from build123d import *

# Parameters (mm, degrees)
SKETCH3_W           = 57.15
SKETCH3_H           = 6.35
BOSS_EXTRUDE2_DEPTH = 50.8
SKETCH4_R           = 5.05
SKETCH4_R_2         = 4.7625
SKETCH4_R_3         = 1.5
SKETCH4_R_4         = 1.984375
CUT_EXTRUDE1_DEPTH  = 6.35


with BuildPart() as part:
    # Sketch3 → Boss-Extrude2 (new body)
    with BuildSketch(Plane.XY):
        with Locations((-92.644673345, -3.175)):
            Rectangle(SKETCH3_W, SKETCH3_H)
    extrude(amount=BOSS_EXTRUDE2_DEPTH)

    # Sketch4 → Cut-Extrude1 (cut)
    with BuildSketch(Plane(origin=(0, 0, 0), x_dir=(1, 0, 0), z_dir=(0, 1, 0))):
        with Locations((-108.519673345, -25.4)):
            Circle(SKETCH4_R)
        with Locations((-79.944673345, -38.1)):
            Circle(SKETCH4_R_2)
        with Locations((-108.519673345, -17.27)):
            Circle(SKETCH4_R_3)
        with Locations((-87.802397451, -30.242275894)):
            Circle(SKETCH4_R_4)
        with Locations((-72.086949239, -30.242275894)):
            Circle(SKETCH4_R_4)
        with Locations((-72.086949239, -45.957724106)):
            Circle(SKETCH4_R_4)
        with Locations((-87.802397451, -45.957724106)):
            Circle(SKETCH4_R_4)
        with Locations((-116.649673345, -25.4)):
            Circle(SKETCH4_R_3)
        with Locations((-100.389673345, -25.4)):
            Circle(SKETCH4_R_3)
        with Locations((-108.519673345, -33.53)):
            Circle(SKETCH4_R_3)
        with Locations((-87.802397451, -4.842275894)):
            Circle(SKETCH4_R_4)
        with Locations((-72.086949239, -4.842275894)):
            Circle(SKETCH4_R_4)
        with Locations((-72.086949239, -20.557724106)):
            Circle(SKETCH4_R_4)
        with Locations((-87.802397451, -20.557724106)):
            Circle(SKETCH4_R_4)
        with Locations((-79.944673345, -12.7)):
            Circle(SKETCH4_R_2)
    extrude(amount=-CUT_EXTRUDE1_DEPTH, mode=Mode.SUBTRACT)


solid = part.part
The model under review builds one solid part; all positions refer to its coordinate system, in mm. Round coordinates to 2 decimals unless told otherwise and drop trailing zeros. Write each loop counter-clockwise with the first axis right and the second up, starting at its lowest first coordinate (ties: lowest second). Pieces come first, ordered by that corner, then holes. Notation, with made-up numbers: (25.5, 37) - (84.5, 37) arc R19 cw to (84.5, 48) - close; hole circle Ø2 at (19.25, -17.75). An arc over 180 degrees is marked (long way). One line per item, written item: value. Start each with the question number.
1. Clearance check with flat-ended pins moving along their axes: P1, Ø5, axis at x = -87.8, z = 30.24, coming from the +Y side; P2, Ø3.5, axis at x = -87.8, z = 45.96, coming from the -Y side. State where each tip first meets the part, or that it passes through.
2. Consider section A-A on z = 12.7. Write out the cut boundary in (x, y), and give its area (3 significant figures).
3. The part is to be moulded in two halves that separate along Z. For faces 1 (the face through (-121.22, -3, 25)), 2 (the face through (-93, -3, 50.8)), 3 (the face through (-85.97, -3.13, 46.72)), say which applies: released by +Z, released by -Z, zero draft, split by the parting line, or undercut.
4. Consider section C-C on x = -89. Write out the cut boundary in (y, z).
5. Consider section B-B on z = 25.4. Write out the cut boundary in (x, y), and give its area (3 significant figures).
6. To check wall thickness, follow L1, parallel to X at y = -2.5, z = 25.4; L2, parallel to X at y = -3.5, z = 46; L3, parallel to Z at x = -88, y = -5.75. State the ranges of each line that lie inside material, in increasing order. Write a range as from..to.
7. Consider section D-D on y = -0.75. State how many separate pieces and enclosed holes the cut face has, and give its area (3 significant figures).
Checks:
1. P1: stops at y = 0
1. P2: passes through
2. outline: (-121.22, -6.35) - (-84.71, -6.35) - (-84.71, 0) - (-121.22, 0) - close; (-75.18, -6.35) - (-64.07, -6.35) - (-64.07, 0) - (-75.18, 0) - close
2. area: 302 mm^2
3. face 1: zero draft
3. face 2: released by +Z
3. face 3: undercut
4. outline: (-6.35, 0) - (0, 0) - (0, 3.26) - (-6.35, 3.26) - close; (-6.35, 6.42) - (0, 6.42) - (0, 18.98) - (-6.35, 18.98) - close; (-6.35, 22.14) - (0, 22.14) - (0, 28.66) - (-6.35, 28.66) - close; (-6.35, 31.82) - (0, 31.82) - (0, 44.38) - (-6.35, 44.38) - close; (-6.35, 47.54) - (0, 47.54) - (0, 50.8) - (-6.35, 50.8) - close
5. outline: (-121.22, -6.35) - (-118.15, -6.35) - (-118.15, 0) - (-121.22, 0) - close; (-115.15, -6.35) - (-113.57, -6.35) - (-113.57, 0) - (-115.15, 0) - close; (-103.47, -6.35) - (-101.89, -6.35) - (-101.89, 0) - (-103.47, 0) - close; (-98.89, -6.35) - (-64.07, -6.35) - (-64.07, 0) - (-98.89, 0) - close
5. area: 261 mm^2
6. L1: x = -121.22..-118.15, -115.15..-113.57, -103.47..-101.89, -98.89..-64.07
6. L2: x = -121.22..-89.79, -85.82..-74.07, -70.1..-64.07
6. L3: z = 0..2.87, 6.82..18.58, 22.53..28.27, 32.22..43.98, 47.93..50.8
7. separate pieces: 1
7. enclosed holes: 15
7. area: 2,550 mm^2
